Work out the finished part from the listing and answer in its coordinate system (mm). Face numbers are marked on the shaded views. A direction names the side the tool comes from. Round coordinates to 2 decimals unless told otherwise and drop trailing zeros. Order: outer loops, then holes, each group sorted by start corner. A loop starts at its lowest first (then second) coordinate and runs counter-clockwise, first axis right, second up. Notation, with made-up numbers: (15.25, 39) - (29.25, 39) arc R10 cw to (29.25, 57) - close; hole circle Ø1 at (-28.75, 51.25). An arc over 180 degrees is marked (long way). Put each result on its own line as item: value.
```python
from build123d import *

# Parameters (mm, degrees)
F0_W     = 41.91
F0_H     = 41.91
F1_DEPTH = 34.036
F2_R     = 1.25
F3_DEPTH = 3.556
F4_R     = 6.35
F5_R     = 10.9982
F6_DEPTH = 1.9812
F7_R     = 2.50063
F8_DEPTH = 24.13


with BuildPart() as f1:
    # F0 (on Top) → F1 (new body)
    with BuildSketch(Plane.XY):
        Rectangle(F0_W, F0_H)
    extrude(amount=F1_DEPTH)

    # F2 (on face) → F3 (cut)
    with BuildSketch(Plane.XY.offset(34.036)):
        with Locations((15.494, -15.494)):
            Circle(F2_R)
        with Locations((15.494, 15.494)):
            Circle(F2_R)
        with Locations((-15.494, 15.494)):
            Circle(F2_R)
        with Locations((-15.494, -15.494)):
            Circle(F2_R)
    extrude(amount=-F3_DEPTH, mode=Mode.SUBTRACT)

    # F4
    f4_edges = [f1.edges().sort_by_distance(p)[0] for p in [
        (-20.955, -20.955, 17.018),
        (20.955, -20.955, 17.018),
        (20.955, 20.955, 17.018),
        (-20.955, 20.955, 17.018),
    ]]
    fillet(f4_edges, radius=F4_R)

    # F5 (on face) → F6 (join)
    with BuildSketch(Plane.XY.offset(34.036)):
        Circle(F5_R)
    extrude(amount=F6_DEPTH)

    # F7 (on face) → F8 (join)
    with BuildSketch(Plane.XY.offset(36.0172)):
        Circle(F7_R)
    extrude(amount=F8_DEPTH)


solid = f1.part
```
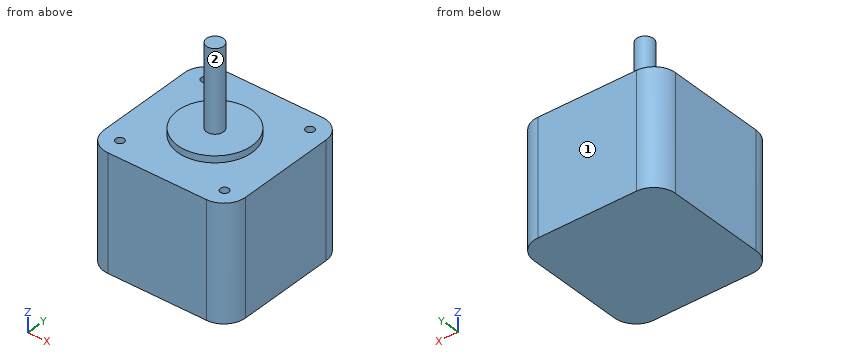
1) For the marked faces 1 and 2, determine the directions among +Z, -Z, +X, -X, +Y, -Y from which every point of the face is accessible in a straight line to the end or side of a thin tool.
Findings below:
face 1: +Z, -Z, +X, -X, +Y
face 2: +Z
2) Straight lines are drawn through the part: L1, parallel to Z at x = 11.5, y = 16; L2, parallel to Z at x = -6, y = 7; L3, parallel to X at y = 15, z = 23.5. For each, find the intervals that lie inside material, in ascending order. Write a range as from..to.
Findings below:
L1: z = 0..34.04
L2: z = 0..36.02
L3: x = -20.94..20.94
3) A cutting plane is placed at D-D on x = 5. Write down the section's boundary in (y, z) (3 decimals).
Findings below:
outline: (-20.955, 0) - (20.955, 0) - (20.955, 34.036) - (9.796, 34.036) - (9.796, 36.017) - (-9.796, 36.017) - (-9.796, 34.036) - (-20.955, 34.036) - close
4) Given pin 1 Ø4 at (x, z) = (-3, 51) entering from -Y; pin 2 Ø0.8 at (x, y) = (15.5, -16) entering from +Z; pin 3 Ø4 at (x, y) = (-15.494, 15.494) entering from +Z, each flat-ended and moving along its own axis, determine where each tip first touches the part or whether it passes through.
Findings below:
pin 1: stops at y = -2.29
pin 2: stops at z = 30.48
pin 3: stops at z = 34.04
5) A cutting plane is placed at A-A on x = 0. Write down the section's boundary in (y, z) (3 decimals), then the cut area to 3 significant figures.
Findings below:
outline: (-20.955, 0) - (20.955, 0) - (20.955, 34.036) - (10.998, 34.036) - (10.998, 36.017) - (2.501, 36.017) - (2.501, 60.147) - (-2.501, 60.147) - (-2.501, 36.017) - (-10.998, 36.017) - (-10.998, 34.036) - (-20.955, 34.036) - close
area: 1,590 mm2
6) A cutting plane is placed at B-B on z = 28.5. Write down the section's boundary in (x, y) (3 decimals).
Findings below:
outline: (-20.955, -14.605) arc R6.35 ccw to (-14.605, -20.955) - (14.605, -20.955) arc R6.35 ccw to (20.955, -14.605) - (20.955, 14.605) arc R6.35 ccw to (14.605, 20.955) - (-14.605, 20.955) arc R6.35 ccw to (-20.955, 14.605) - close
